```python
from build123d import *

# Parameters (mm, degrees)
F0_R     = 13.5
F0_R_2   = 7.5
F1_DEPTH = 5.08


with BuildPart() as f1:
    # F0 (on Front) → F1 (new body)
    with BuildSketch(Plane.XZ):
        with BuildLine():
            Line((5.08, 0), (178.75, 0))
            ThreePointArc((178.75, 0), (204.15, 25.4), (178.75, 50.8))
            Line((178.75, 50.8), (5.08, 50.8))
            Line((5.08, 50.8), (5.08, 40.8))
            Line((5.08, 40.8), (0, 40.8))
            Line((0, 40.8), (0, 30.4))
            Line((0, 30.4), (5.08, 30.4))
            Line((5.08, 30.4), (5.08, 20.4))
            Line((5.08, 20.4), (0, 20.4))
            Line((0, 20.4), (0, 10))
            Line((0, 10), (5.08, 10))
            Line((5.08, 10), (5.08, 0))
        make_face()
        with Locations((97.259023, 25.8)):
            Circle(F0_R, mode=Mode.SUBTRACT)
        with Locations((178.75, 25.4)):
            Circle(F0_R_2, mode=Mode.SUBTRACT)
    extrude(amount=F1_DEPTH)


solid = f1.part
```
The model under review builds one solid part; all positions refer to its coordinate system, in mm. A direction names the side the tool comes from. Give positions to 0.01 mm unless a question says otherwise; leave off trailing zeros. Write each loop counter-clockwise with the first axis right and the second up, starting at its lowest first coordinate (ties: lowest second). Pieces come first, ordered by that corner, then holes. Notation, with made-up numbers: (-23.75, -16) -> (-7.75, -16) arc R25 cw to (-7.75, -2) -> close; hole circle Ø11 at (-8, -15.75). An arc over 180 degrees is marked (long way). Put each result on its own line as item: value.
(1) The part is to be moulded in two halves that separate along X. For faces 1 (the flat face through (3, -3, 10)), 2 (the flat face through (0, -3, 15)), 3 (the cylindrical face through (185.68, -2.5, 22.53)), say which applies: pulls with the +X half, pulls with the -X half, needs draft (parallel to the pull), parting line crosses it, or undercut.
Results are:
face 1: needs draft
face 2: pulls with the -X half
face 3: undercut
(2) Tool access review of faces 4 (the flat face through (5.08, -3, 5)), 5 (the flat face through (101, 0, 9)), 6 (the flat face through (3, -3, 40.8)), 7 (the flat face through (3, -3, 30.4)): name each direction out of +Z, -Z, +X, -X, +Y, -Y from which nothing blocks a thin tool from reaching the whole face with its end or side.
Results are:
face 4: -Z, -X, +Y, -Y
face 5: +Z, -Z, +X, -X, +Y
face 6: +Z, -X, +Y, -Y
face 7: -X, +Y, -Y
(3) We need section A-A, the plane y = -1.2. Give the boundary of the cut face in (x, z), and give its area (3 significant figures).
Results are:
outline: (0, 10) -> (5.08, 10) -> (5.08, 0) -> (178.75, 0) arc R25.4 ccw to (178.75, 50.8) -> (5.08, 50.8) -> (5.08, 40.8) -> (0, 40.8) -> (0, 30.4) -> (5.08, 30.4) -> (5.08, 20.4) -> (0, 20.4) -> close; hole circle Ø27 at (97.26, 25.8); hole circle Ø15 at (178.75, 25.4)
area: 9,190 mm²
(4) We need section D-D, the plane z = 8. Give the boundary of the cut face in (x, y).
Results are:
outline: (5.08, -5.08) -> (197.25, -5.08) -> (197.25, 0) -> (5.08, 0) -> close
(5) To check wall thickness, follow probe 1 along Z at (x, y) = (178.75, -2.7); probe 2 along X at (y, z) = (-1.4, 27); probe 3 along X at (y, z) = (-4.35, 21). State the ranges of each line that lie inside material, in increasing order. Write a range as from..to.
Results are:
probe 1: 0..17.9, 32.9..50.8
probe 2: 5.08..83.81, 110.71..171.42, 186.08..204.1
probe 3: 5.08..84.64, 109.88..172.68, 184.82..203.77
(6) We need section B-B, the plane z = 35.5. Give the boundary of the cut face in (x, y).
Results are:
outline: (0, -5.08) -> (87.87, -5.08) -> (87.87, 0) -> (0, 0) -> close; (106.65, -5.08) -> (202.06, -5.08) -> (202.06, 0) -> (106.65, 0) -> close
(7) For pin 1 Ø2.5 at (x, y) = (2, -3.5) entering from -Z; pin 2 Ø1.5 at (y, z) = (-3, 4) entering from -X; pin 3 Ø1.5 at (x, y) = (3, -2.5) entering from +Z, all flat-tipped, find the tip position at first contact; note any pin that passes through.
Results are:
pin 1: z = 10
pin 2: x = 5.08
pin 3: z = 40.8
(8) We need section C-C, the plane x = 183. Give the boundary of the cut face in (y, z), and give its area (3 significant figures).
Results are:
outline: (-5.08, 0.36) -> (0, 0.36) -> (0, 19.22) -> (-5.08, 19.22) -> close; (-5.08, 31.58) -> (0, 31.58) -> (0, 50.44) -> (-5.08, 50.44) -> close
area: 192 mm²
